```python
from build123d import *

# Parameters (mm, degrees)
BOSS_EXTRUDE1_DEPTH = 18
CHAMFER1_START      = -1
CHAMFER1_OUTLINE_W  = 28
CHAMFER1_OUTLINE_H  = 793
CHAMFER1_DEPTH      = 13.727922061


with BuildPart() as part:
    # Sketch1 → Boss-Extrude1 (new body)
    with BuildSketch(Plane.XY):
        with BuildLine():
            Line((278.994949366, 786.142135624), (265.710678119, 772.857864376))
            ThreePointArc((265.710678119, 772.857864376), (259.222211142, 768.52240935), (251.568542495, 767))
            Line((251.568542495, 767), (191.568542495, 767))
            ThreePointArc((191.568542495, 767), (183.914873848, 768.52240935), (177.426406871, 772.857864376))
            Line((177.426406871, 772.857864376), (164.142135624, 786.142135624))
            ThreePointArc((164.142135624, 786.142135624), (157.653668647, 790.47759065), (150, 792))
            Line((150, 792), (0, 792))
            Line((0, 792), (0, 0))
            Line((0, 0), (430, 0))
            Line((430, 0), (430, 792))
            Line((430, 792), (293.13708499, 792))
            ThreePointArc((293.13708499, 792), (285.483416343, 790.47759065), (278.994949366, 786.142135624))
        make_face()
    extrude(amount=BOSS_EXTRUDE1_DEPTH)

    # Chamfer1: read off the stored shape, not the designer's step
    # Chamfer1 outline → Chamfer1 (cut)
    with BuildSketch(Plane(origin=(0, 0, 0), x_dir=(0.7071067811865471, 0, -0.707106781186548), z_dir=(0.707106781186548, 0, 0.707106781186547)).offset(CHAMFER1_START)):
        with Locations((0, 395.5)):
            Rectangle(CHAMFER1_OUTLINE_W, CHAMFER1_OUTLINE_H)
    extrude(amount=CHAMFER1_DEPTH, mode=Mode.SUBTRACT)


solid = part.part
```
Geometry: final body of the model. Coordinates: model frame, mm. A direction names the side the tool comes from. Round coordinates to 2 decimals unless told otherwise and drop trailing zeros. Loops run counter-clockwise (first coordinate to the right, second up) from the corner with the lowest first, then second, coordinate; pieces in that order, holes last.
Item 1: Section A-A, the plane z = 5. Output: boundary loops of the cut face in (x, y).
Checked values:
outline: (13, 0) - (430, 0) - (430, 792) - (293.14, 792) arc R20 ccw to (278.99, 786.14) - (265.71, 772.86) arc R20 cw to (251.57, 767) - (191.57, 767) arc R20 cw to (177.43, 772.86) - (164.14, 786.14) arc R20 ccw to (150, 792) - (13, 792) - close
Item 2: Mould query, pull axis X, two halves, no side actions, for faces 3 (the cylindrical face through (285.59, 790.52, 8.87)), 4 (the flat face through (222, 767, 9)), 5 (the flat face through (9, 402, 9)), 6 (the flat face through (221, 402, 0)). Classes: released by +X, released by -X, zero draft, split by the parting line, or undercut.
Checked values:
face 3: undercut
face 4: undercut
face 5: released by -X
face 6: zero draft
Item 3: Section C-C, the plane y = 431.5. Output: boundary loops of the cut face in (x, z).
Checked values:
outline: (0, 18) - (18, 0) - (430, 0) - (430, 18) - close
Item 4: Reachability of faces 1 (the flat face through (76, 792, 9)), 2 (the cylindrical face through (184.02, 768.48, 8.87)) from +Z, -Z, +X, -X, +Y, -Y: full face, straight path, thin tool, end or side. Return the list, or none.
Checked values:
face 1: +Z, -Z, +X, -X, +Y
face 2: +Z, -Z, +Y
Item 5: Section B-B, the plane x = 205. Output: boundary loops of the cut face in (y, z).
Checked values:
outline: (0, 0) - (767, 0) - (767, 18) - (0, 18) - close
Item 6: Line query: L1, parallel to Y at x = 243, z = 11; L2, parallel to Y at x = 166.5, z = 1.5; L3, parallel to X at y = 459, z = 8.25. Output: solid intervals per line, ascending.
Checked values:
L1: y = 0 to 767
L2: y = 0 to 783.78
L3: x = 9.75 to 430
